Here's how the part is built. I have some questions about the finished solid (model axes, mm). A direction names the side the tool comes from. Round coordinates to 2 decimals unless told otherwise and drop trailing zeros. Order: outer loops, then holes, each group sorted by start corner. A loop starts at its lowest first (then second) coordinate and runs counter-clockwise, first axis right, second up. Notation, with made-up numbers: (67, -25) - (74, -25) arc R20 ccw to (74, -3) - close; hole circle Ø6 at (66, -9). An arc over 180 degrees is marked (long way). Answer as a JSON object with one key per item and string values.
Autodesk Inventor part; units mm, degrees
ref_plane "YZ Plane" through (0, 0, 0) normal (1, 0, 0) x (0, 1, 0)
ref_plane "XZ Plane" through (0, 0, 0) normal (0, 1, 0) x (-1, 0, 0)
ref_plane "XY Plane" through (0, 0, 0) normal (0, 0, 1) x (1, 0, 0)
sketch "Sketch1" plane through (0, 0, 0) normal (0, 1, 0) x (-1, 0, 0)
  line L0 (0, 0) -> (0, 10)
  line L1 (0, 10) -> (42.6685, 10)
  line L2 (0, 0) -> (38.0054, 0)
  line L3 (41.8356, -1.7861) -> (83.8302, -51.8333)
  line L4 (85, -55.0472) -> (85, -60.1449)
  line L5 (90, -65.1449) -> (90, -65.1449)
  line L6 (95, -60.1449) -> (95, -51.4075)
  line L7 (93.8302, -48.1936) -> (46.4987, 8.2139)
  arc A0 (45.5995, 9.2856) -> (44.0674, 10) centre (44.0674, 8) ccw
  arc A1 (41.8356, -1.7861) -> (38.0054, 0) centre (38.0054, -5) ccw
  arc A2 (85, -55.0472) -> (83.8302, -51.8333) centre (80, -55.0472) ccw
  arc A3 (95, -51.4075) -> (93.8302, -48.1936) centre (90, -51.4075) ccw
  arc A4 (46.4987, 8.2139) -> (42.6685, 10) centre (42.6685, 5) ccw
  arc A5 (90, -65.1449) -> (95, -60.1449) centre (90, -60.1449) ccw
  arc A6 (85, -60.1449) -> (90, -65.1449) centre (90, -60.1449) ccw
  point P0 (85, -65.1449)
  point P1 (95, -65.1449)
  point P2 (45, 10)
  point P3 (90, -65.1449)
  dimension "d1" = 130
  dimension "d2" = 140
  dimension "d3" = 45
  dimension "d4" = 50
  dimension "d5" = 10
  dimension "d6" = 10
  dimension "d7" = 10
  dimension "d8" = 2
  dimension "d9" = 5
extrude "Extrusion1" add sketch "Sketch1" along normal blind 3
sketch "Sketch2" plane through (0, 3, 0) normal (0, 1, 0) x (1, 0, 0)
  line L0 (0, -10) -> (0, 0)
  line L1 (0, -5) -> (-25.3234, -5) construction
  arc A0 (-85, 60.1449) -> (-95, 60.1449) centre (-90, 60.1449) ccw
  point P0 (-6.55, -5)
  dimension "d19" = 6.55
hole "Hole1" at (-6.55, 3, 5) at (-90, 3, -60.1449) direction (0, -1, 0) diameter 3.2 end through all
mirror "Mirror1" about plane through (0, 0, 0) normal (1, 0, 0) of "Extrusion1", "Hole1"
properties part number "Claw1" material "Copper, Cast"
1. Imagine slicing it at A-A (y = 1.95). List the corners of the cut face in (x, z) for me, plus the area to 3 significant figures.
Responses:
{"outline": "(-95, -60.14) arc R5 ccw to (-85, -60.14) - (-85, -55.05) arc R5 cw to (-83.83, -51.83) - (-41.84, -1.79) arc R5 cw to (-38.01, 0) - (38.01, 0) arc R5 cw to (41.84, -1.79) - (83.83, -51.83) arc R5 cw to (85, -55.05) - (85, -60.14) arc R5 ccw to (95, -60.14) - (95, -51.41) arc R5 ccw to (93.83, -48.19) - (46.5, 8.21) arc R5 ccw to (42.67, 10) - (-42.67, 10) arc R5 ccw to (-46.5, 8.21) - (-93.83, -48.19) arc R5 ccw to (-95, -51.41) - close; hole circle Ø3.2 at (-90, -60.14); hole circle Ø3.2 at (-6.55, 5); hole circle Ø3.2 at (6.55, 5); hole circle Ø3.2 at (90, -60.14)", "area": "2,550 mm2"}
2. Imagine slicing it at B-B (z = -6). List the corners of the cut face in (x, y) for me, plus the area to 3 significant figures.
Responses:
{"outline": "(-58.43, 0) - (-45.37, 0) - (-45.37, 3) - (-58.43, 3) - close; (45.37, 0) - (58.43, 0) - (58.43, 3) - (45.37, 3) - close", "area": "78.3 mm2"}
3. For faces 1 (the face through (89.93, 1.479, -61.743)), 2 (the face through (63.127, 1.479, -27.16)), which set-ups out of +Z, -Z, +X, -X, +Y, -Y let a thin tool reach every point of the face, with its end or its side?
Responses:
{"face 1": "+Y, -Y", "face 2": "-Z, +Y, -Y"}
4. For P1, Ø2.5, axis at x = -6.55, z = 5, coming from the -Y side; P2, Ø5, axis at x = -90, z = -60.14, coming from the +Y side; P3, Ø1.5, axis at y = 1, z = -15.5, coming from the -X side; P4, Ø1.5, axis at y = 1.5, z = 0.5, coming from the -X side, each with a flat end and sliding along its axis, tell me the tip position at first contact or that it passes through.
Responses:
{"P1": "through", "P2": "y = 3", "P3": "x = -67.03", "P4": "x = -53.6"}
5. Thinking about a two-plate mould opening in X: for faces 3 (the face through (14.5, 3, 0.4)), 4 (the face through (-70.496, 1.479, -20.385)), 5 (the face through (-62.54, 1.48, -26.46)), which applies, pulls with the +X half, pulls with the -X half, needs draft (parallel to the pull), parting line crosses it, or undercut?
Responses:
{"face 3": "needs draft", "face 4": "pulls with the -X half", "face 5": "undercut"}
6. Imagine slicing it at D-D (x = 63.5). List the corners of the cut face in (y, z) for me.
Responses:
{"outline": "(0, -27.6) - (3, -27.6) - (3, -12.05) - (0, -12.05) - close"}
7. If I drill on L1, parallel to X at y = 1.15, z = 5; L2, parallel to Z at x = 6.55, y = 1.3; L3, parallel to Z at x = -32.5, y = 2.7, over which ranges is the centre line in solid material (lowest first)? Write a range as [from, to].
Responses:
{"L1": "[-49.2, -8.15], [-4.95, 4.95], [8.15, 49.2]", "L2": "[0, 3.4], [6.6, 10]", "L3": "[0, 10]"}
8. Imagine slicing it at C-C (x = 17). List the corners of the cut face in (y, z) for me, plus the area to 3 significant figures.
Responses:
{"outline": "(0, 0) - (3, 0) - (3, 10) - (0, 10) - close", "area": "30.0 mm2"}
